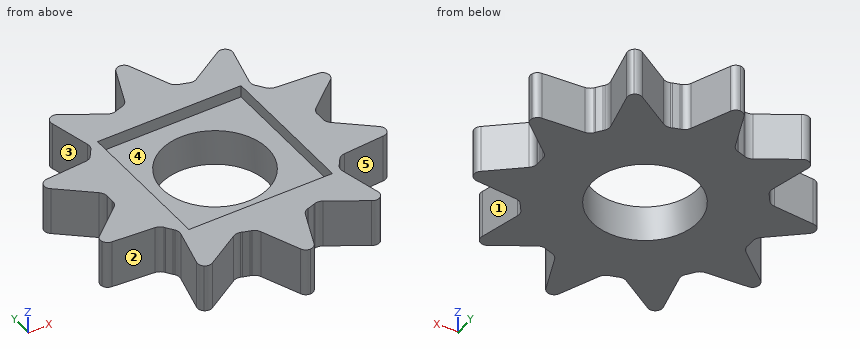
from build123d import *

# Parameters (mm, degrees)
F1_DEPTH        = 1
F1_COPIES_COUNT = 10
F3_W            = 3
F3_H            = 3
F4_DEPTH        = 0.25
F5_DEPTH        = 1
F6_DEPTH        = 0.25
F7_R            = 1.1
F8_DEPTH        = 1.31


# Not quite as in the source:
# - ends of sketch curves that miss each other by under 0.0002 mm in the source are joined
# - a feature of the source that left no trace in its solid (it failed there, or was rolled back) is left out
# - a pattern or mirror of a feature is missing from the dataset's text; its kind, count and spacing are read off the source's solid


with BuildPart() as f1:
    # F0 (on Top) → F1 (new body)
    with BuildSketch(Plane.XY):
        with BuildLine():
            ThreePointArc((0.581444512, 2.1217733808), (0.2933415776, 2.1803556405), (0, 2.2))
            ThreePointArc((0, 2.2), (-0.2933416878, 2.1803556256), (-0.5814447265, 2.121773322))
            ThreePointArc((-0.5814447265, 2.121773322), (-0.5968372157, 2.1167523736), (-0.6125853979, 2.1129929319))
            ThreePointArc((-0.6125853979, 2.1129929319), (-1.3214219849, -1.7589326132), (2.2, 0))
            ThreePointArc((2.2, 0), (1.7589325969, 1.3214220066), (0.612585346, 2.112992947))
            ThreePointArc((0.6125853416, 2.1129929319), (0.5968370782, 2.1167523965), (0.581444512, 2.1217733808))
        make_face()
        with BuildLine():
            ThreePointArc((0.6, 0.8), (0, -1), (-0.6, 0.8))
            Line((-0.6, 0.8), (0, 0.8))
            Line((0, 0.8), (0.6, 0.8))
        make_face(mode=Mode.SUBTRACT)
        with BuildLine():
            ThreePointArc((-0.5814447265, 2.121773322), (-0.2933416878, 2.1803556256), (0, 2.2))
            Line((0, 2.2), (0, 2.8273255734))
            ThreePointArc((0, 2.8273255734), (-0.1215931939, 2.889819495), (-0.1419835484, 3.0250031792))
            Line((-0.1419835484, 3.0250031792), (-0.4660251262, 2.233467269))
            ThreePointArc((-0.4660251262, 2.233467269), (-0.5120300634, 2.1655250062), (-0.5814447265, 2.121773322))
        make_face()
        with BuildLine():
            Line((0, 2.8273255734), (0, 2.2))
            ThreePointArc((0, 2.2), (0.2933415776, 2.1803556405), (0.581444512, 2.1217733808))
            ThreePointArc((0.581444512, 2.1217733808), (0.5119904355, 2.165563311), (0.4659834267, 2.2335690598))
            Line((0.4659834267, 2.2335690598), (0.1424618925, 3.0249932315))
            ThreePointArc((0.1424618925, 3.0249932315), (0.1482808399, 3.0014743175), (0.1502375048, 2.9773253853))
            ThreePointArc((0.1502375048, 2.9773253853), (0.1062195181, 2.8711754307), (0, 2.8273255734))
        make_face()
        with BuildLine():
            ThreePointArc((-0.1419835484, 3.0250031792), (-0.1215931939, 2.889819495), (0, 2.8273255734))
            Line((0, 2.8273255734), (0, 3.1273251973))
            ThreePointArc((0, 3.1273251973), (-0.0874611784, 3.0990173775), (-0.1419835484, 3.0250031792))
        make_face()
        with BuildLine():
            Line((0, 3.1273251973), (0, 2.8273255734))
            ThreePointArc((0, 2.8273255734), (0.1062195181, 2.8711754307), (0.1502375048, 2.9773253853))
            ThreePointArc((0.1502375048, 2.9773253853), (0.1482808399, 3.0014743175), (0.1424618925, 3.0249932315))
            ThreePointArc((0.1424618925, 3.0249932315), (0.0877476558, 3.0991530237), (0, 3.1273251973))
        make_face()
        with BuildLine():
            ThreePointArc((0.612585346, 2.112992947), (0.5970310708, 2.1174404125), (0.581444512, 2.1217733808))
            ThreePointArc((0.581444512, 2.1217733808), (0.5968370782, 2.1167523965), (0.6125853416, 2.1129929319))
        make_face()
        with BuildLine():
            ThreePointArc((-0.6125853979, 2.1129929319), (-0.5968372157, 2.1167523736), (-0.5814447265, 2.121773322))
            ThreePointArc((-0.5814447265, 2.121773322), (-0.5970312038, 2.117440375), (-0.6125853979, 2.1129929319))
        make_face()
    extrude(amount=F1_DEPTH)

    # F1_copies: F1 ×10 about axis
    f1_copies_axis = Axis((0, 0, 0), (0, 0, 1))


with BuildPart() as f1_1:
    add(f1.part)
    for i in range(1, F1_COPIES_COUNT):
        add(f1.part.rotate(f1_copies_axis, i * 360 / F1_COPIES_COUNT))

    # F3 (on face) → F4 (cut)
    with BuildSketch(Plane.XY.offset(1)):
        Rectangle(F3_W, F3_H)
    extrude(amount=-F4_DEPTH, mode=Mode.SUBTRACT)

    # F0 (on Top) → F5 (join)
    with BuildSketch(Plane.XY):
        with BuildLine():
            ThreePointArc((0.581444512, 2.1217733808), (0.2933415776, 2.1803556405), (0, 2.2))
            ThreePointArc((0, 2.2), (-0.2933416878, 2.1803556256), (-0.5814447265, 2.121773322))
            ThreePointArc((-0.5814447265, 2.121773322), (-0.5968372157, 2.1167523736), (-0.6125853979, 2.1129929319))
            ThreePointArc((-0.6125853979, 2.1129929319), (-1.3214219849, -1.7589326132), (2.2, 0))
            ThreePointArc((2.2, 0), (1.7589325969, 1.3214220066), (0.612585346, 2.112992947))
            ThreePointArc((0.6125853416, 2.1129929319), (0.5968370782, 2.1167523965), (0.581444512, 2.1217733808))
        make_face()
        with BuildLine():
            ThreePointArc((0.6, 0.8), (0, -1), (-0.6, 0.8))
            Line((-0.6, 0.8), (0, 0.8))
            Line((0, 0.8), (0.6, 0.8))
        make_face(mode=Mode.SUBTRACT)
        with BuildLine():
            ThreePointArc((-0.5814447265, 2.121773322), (-0.2933416878, 2.1803556256), (0, 2.2))
            Line((0, 2.2), (0, 2.8273255734))
            ThreePointArc((0, 2.8273255734), (-0.1215931939, 2.889819495), (-0.1419835484, 3.0250031792))
            Line((-0.1419835484, 3.0250031792), (-0.4660251262, 2.233467269))
            ThreePointArc((-0.4660251262, 2.233467269), (-0.5120300634, 2.1655250062), (-0.5814447265, 2.121773322))
        make_face()
        with BuildLine():
            Line((0, 2.8273255734), (0, 2.2))
            ThreePointArc((0, 2.2), (0.2933415776, 2.1803556405), (0.581444512, 2.1217733808))
            ThreePointArc((0.581444512, 2.1217733808), (0.5119904355, 2.165563311), (0.4659834267, 2.2335690598))
            Line((0.4659834267, 2.2335690598), (0.1424618925, 3.0249932315))
            ThreePointArc((0.1424618925, 3.0249932315), (0.1482808399, 3.0014743175), (0.1502375048, 2.9773253853))
            ThreePointArc((0.1502375048, 2.9773253853), (0.1062195181, 2.8711754307), (0, 2.8273255734))
        make_face()
        with BuildLine():
            ThreePointArc((-0.1419835484, 3.0250031792), (-0.1215931939, 2.889819495), (0, 2.8273255734))
            Line((0, 2.8273255734), (0, 3.1273251973))
            ThreePointArc((0, 3.1273251973), (-0.0874611784, 3.0990173775), (-0.1419835484, 3.0250031792))
        make_face()
        with BuildLine():
            Line((0, 3.1273251973), (0, 2.8273255734))
            ThreePointArc((0, 2.8273255734), (0.1062195181, 2.8711754307), (0.1502375048, 2.9773253853))
            ThreePointArc((0.1502375048, 2.9773253853), (0.1482808399, 3.0014743175), (0.1424618925, 3.0249932315))
            ThreePointArc((0.1424618925, 3.0249932315), (0.0877476558, 3.0991530237), (0, 3.1273251973))
        make_face()
        with BuildLine():
            ThreePointArc((0.612585346, 2.112992947), (0.5970310708, 2.1174404125), (0.581444512, 2.1217733808))
            ThreePointArc((0.581444512, 2.1217733808), (0.5968370782, 2.1167523965), (0.6125853416, 2.1129929319))
        make_face()
        with BuildLine():
            ThreePointArc((-0.6125853979, 2.1129929319), (-0.5968372157, 2.1167523736), (-0.5814447265, 2.121773322))
            ThreePointArc((-0.5814447265, 2.121773322), (-0.5970312038, 2.117440375), (-0.6125853979, 2.1129929319))
        make_face()
    extrude(amount=F5_DEPTH)

    # F3 (on face) → F6 (cut)
    with BuildSketch(Plane.XY.offset(1)):
        Rectangle(F3_W, F3_H)
        Polygon((-0.259935757, 0.8), (0.259935757, 0.8), (0.6805206467, 0.494427191), (0.8411697794, 0), (0.6805206467, -0.494427191), (0.259935757, -0.8), (-0.259935757, -0.8), (-0.6805206467, -0.494427191), (-0.8411697794, 0), (-0.6805206467, 0.494427191), align=None, mode=Mode.SUBTRACT)
    extrude(amount=-F6_DEPTH, mode=Mode.SUBTRACT)

    # F7 (on face) → F8 (cut, symmetric)
    with BuildSketch(Plane.XY.offset(1)):
        Circle(F7_R)
    extrude(amount=F8_DEPTH, both=True, mode=Mode.SUBTRACT)


solid = f1_1.part
The listing builds one solid part. Answer for the finished solid, in the listing's coordinates (mm). Face numbers are marked on the shaded views. A direction names the side the tool comes from. Coordinates: 2 decimals unless noted, no trailing zeros. Write each loop counter-clockwise with the first axis right and the second up, starting at its lowest first coordinate (ties: lowest second). Pieces come first, ordered by that corner, then holes. Notation, with made-up numbers: (35.25, 61) - (72.25, 61) arc R15 cw to (72.25, 86) - close; hole circle Ø6 at (-24.75, 1). An arc over 180 degrees is marked (long way). Return JSON: item names as keys, results as strings.
1. Consider line 1 along Y through (x, z) = (0, 0.25); line 2 along X through (y, z) = (2.25, 0.25); line 3 along X through (y, z) = (2.5, 0.2). Determine where each line is inside the solid, lowest interval first.
Final values:
{"line 1": "-3.13 to -1.1, 1.1 to 3.13", "line 2": "-1.87 to -1.21, -0.46 to 0.46, 1.21 to 1.87", "line 3": "-1.87 to -1.61, -0.36 to 0.36, 1.61 to 1.87"}
2. The part is cut by section A-A on x = 0.85. Determine the outline of the cut face in (y, z).
Final values:
{"outline": "(-2.05, 0) - (-0.7, 0) - (-0.7, 0.75) - (-1.5, 0.75) - (-1.5, 1) - (-2.05, 1) - close; (0.7, 0) - (2.05, 0) - (2.05, 1) - (1.5, 1) - (1.5, 0.75) - (0.7, 0.75) - close"}
3. For a pull along X with two mould halves and no side action, classify the marked faces 3, 4 and 5 as +X half, -X half, draft (parallel to the pull), parting line (faces both ways), or undercut.
Final values:
{"face 3": "-X half", "face 4": "undercut", "face 5": "+X half"}
4. Which of the six approach directions +Z, -Z, +X, -X, +Y, -Y give full straight-line access (tool end or side, diameter ignored) to the marked faces 1 and 2?
Final values:
{"face 1": "+Z, -Z, +X", "face 2": "+Z, -Z, -X, -Y"}
5. This flat-tipped pin is pushed along its axis until it touches: pin 1 Ø1 at (x, y) = (0.5, 0.5) entering from +Z. Where does it stop, or does it pass through?
Final values:
{"pin 1": "z = 0.75"}
6. The part is cut by section B-B on y = 0.5. Determine the outline of the cut face in (x, z), then the cut area to 3 significant figures.
Final values:
{"outline": "(-2.57, 0) - (-0.98, 0) - (-0.98, 0.75) - (-1.5, 0.75) - (-1.5, 1) - (-2.57, 1) - close; (0.98, 0) - (2.57, 0) - (2.57, 1) - (1.5, 1) - (1.5, 0.75) - (0.98, 0.75) - close", "area": "2.91 mm^2"}
